Check sheet for the modelled part. Datum: model origin and axes. Units: mm. A direction names the side the tool comes from. Round coordinates to 2 decimals unless told otherwise and drop trailing zeros. Loops run counter-clockwise (first coordinate to the right, second up) from the corner with the lowest first, then second, coordinate; pieces in that order, holes last. Notation, with made-up numbers: (88.25, -36.5) - (139.25, -36.5) arc R8 ccw to (139.25, -26.5) - close; hole circle Ø5 at (40, 18). An arc over 180 degrees is marked (long way). Put each result on its own line as item: value.
Autodesk Inventor part; units mm, degrees
ref_plane "YZ Plane" through (0, 0, 0) normal (1, 0, 0) x (0, 1, 0)
ref_plane "XZ Plane" through (0, 0, 0) normal (0, 1, 0) x (-1, 0, 0)
ref_plane "XY Plane" through (0, 0, 0) normal (0, 0, 1) x (1, 0, 0)
sketch "Sketch1" plane through (0, 0, 0) normal (0, 0, 1) x (1, 0, 0)
  line L0 (-13, 12) -> (13, 12)
  line L1 (13, 12) -> (13, -12)
  line L2 (13, -12) -> (-13, -12)
  line L3 (-13, -12) -> (-13, 12)
  line L4 (-13, 3.25) -> (-15, 3.25)
  line L5 (-15, 3.25) -> (-15, -3.25)
  line L6 (-15, -3.25) -> (-13, -3.25)
  line L7 (-13, -3.25) -> (-13, 3.25)
  line L8 (13, 3.25) -> (15, 3.25)
  line L9 (15, 3.25) -> (15, -3.25)
  line L10 (15, -3.25) -> (13, -3.25)
  line L11 (13, -3.25) -> (13, 3.25)
  line L12 (-25.4, 25.4) -> (25.4, 25.4)
  line L13 (25.4, 25.4) -> (25.4, -25.4)
  line L14 (25.4, -25.4) -> (-25.4, -25.4)
  line L15 (-25.4, -25.4) -> (-25.4, 25.4)
  circle A0 centre (0, 0) radius 7.1437
  circle A1 centre (-3, 12) radius 1.5
  line L16 (-13, 8) -> (-9, 12)
  line L17 (9, 12) -> (13, 8)
  line L18 (13, -8) -> (9, -12)
  line L19 (-13, -8) -> (-9, -12)
  point P0 (-14, 3.25)
  point P1 (14, 3.25)
  point P2 (-14, -3.25)
  point P3 (14, -3.25)
  point P4 (-20.32, 20.32)
  point P5 (20.32, 20.32)
  point P6 (20.32, -20.32)
  point P7 (-20.32, -20.32)
  dimension "d0" = 24
  dimension "d1" = 12
  dimension "d2" = 26
  dimension "d3" = 13
  dimension "d4" = 2
  dimension "d5" = 6.5
  dimension "d6" = 3.25
  dimension "d7" = 2
  dimension "d8" = 14.2875
  dimension "d9" = 50.8
  dimension "d10" = 25.4
  dimension "d11" = 50.8
  dimension "d12" = 25.4
  dimension "d13" = 3
  dimension "d14" = 10
  dimension "d15" = 4
  dimension "d16" = 4
  dimension "d17" = 4
  dimension "d18" = 4
  dimension "d19" = 4
  dimension "d20" = 5.08
  dimension "d21" = 5.08
  dimension "d22" = 5.08
  dimension "d23" = 5.08
  dimension "d34" = 40.64
  dimension "d35" = 40.64
extrude "Extrusion1" add sketch "Sketch1" against normal blind 18.2626 contours L0 L16 L3 | L0 L1 L17 | L19 L2 L3 | L18 L1 L2 | L12 L13 L14 L15
fillet "Fillet1" radius 3.175 4 edges at (-13, -3.25, -9.1313) (-13, 3.25, -9.1313) (13, 3.25, -9.1313) (13, -3.25, -9.1313)
hole "Hole1" at (-20.32, 20.32, 0) at (20.32, 20.32, 0) at (20.32, -20.32, 0) at (-20.32, -20.32, 0) direction (0, 0, -1) diameter 4.572 end through all
thread "Thread1"
thread "Thread2"
thread "Thread3"
thread "Thread4"
equation "\"d7\" = d4"
equation "\"d16\" = d15"
equation "\"d17\" = d15"
equation "\"d18\" = d15"
equation "\"d19\" = d15"
properties part number "BD gearbox mount block"
Item 1: Thickness scan on line 1 (X direction, y = 20.32, z = -5.75); line 2 (X direction, y = 0, z = -9). Record the ranges inside material, lowest first. Write a range as from..to.
Filled sheet:
line 1: -25.4..-22.61, -18.03..18.03, 22.61..25.4
line 2: -25.4..-15, 15..25.4
Item 2: Section check B-B on y = -9.5. Enter the section's corners in (x, z).
Filled sheet:
outline: (-25.4, -18.26) - (-11.5, -18.26) - (-11.5, 0) - (-25.4, 0) - close; (11.5, -18.26) - (25.4, -18.26) - (25.4, 0) - (11.5, 0) - close
Item 3: Section check A-A on x = -20.32. Enter the section's corners in (y, z).
Filled sheet:
outline: (-25.4, -18.26) - (-22.61, -18.26) - (-22.61, 0) - (-25.4, 0) - close; (-18.03, -18.26) - (18.03, -18.26) - (18.03, 0) - (-18.03, 0) - close; (22.61, -18.26) - (25.4, -18.26) - (25.4, 0) - (22.61, 0) - close
Item 4: Section check C-C on z = -7. Enter the section's corners in (x, y) (3 decimals), then the cut area to 3 significant figures.
Filled sheet:
outline: (-25.4, -25.4) - (25.4, -25.4) - (25.4, 25.4) - (-25.4, 25.4) - close; hole circle Ø4.572 at (-20.32, -20.32); hole circle Ø4.572 at (-20.32, 20.32); hole (-15, -3.25) arc R3.175 cw to (-13, -6.2) - (-13, -8) - (-9, -12) - (9, -12) - (13, -8) - (13, -6.2) arc R3.175 cw to (15, -3.25) - (15, 3.25) arc R3.175 cw to (13, 6.2) - (13, 8) - (9, 12) - (-1.5, 12) arc R1.5 ccw to (-4.5, 12) - (-9, 12) - (-13, 8) - (-13, 6.2) arc R3.175 cw to (-15, 3.25) - close; hole circle Ø4.572 at (20.32, -20.32); hole circle Ø4.572 at (20.32, 20.32)
area: 1,890 mm²
Item 5: Tool access check on faces 1 (the cylindrical face through (13.53, 4.44, -9)), 2 (the flat face through (-25.4, 0, -9)). Record the directions out of +Z, -Z, +X, -X, +Y, -Y that give a thin tool (end or side, any length) a straight path to the whole face; none if there is none.
Filled sheet:
face 1: +Z, -Z
face 2: +Z, -Z, -X, +Y, -Y
Item 6: Release check for a two-part mould opening along Y. For faces 3 (the cylindrical face through (-13.56, 4.4, -9)), 4 (the flat face through (25.4, 0, -9)) record: +Y half, -Y half, draft (parallel to the pull), parting line (faces both ways), or undercut.
Filled sheet:
face 3: undercut
face 4: draft
Item 7: Section check D-D on x = -3. Enter the section's corners in (y, z).
Filled sheet:
outline: (-25.4, -18.26) - (-12, -18.26) - (-12, 0) - (-25.4, 0) - close; (13.5, -18.26) - (25.4, -18.26) - (25.4, 0) - (13.5, 0) - close
